Work out the finished part from the listing and answer in its coordinate system (mm). Face numbers are marked on the shaded views. A direction names the side the tool comes from. Give positions to 0.01 mm unless a question says otherwise; leave off trailing zeros. Loops run counter-clockwise (first coordinate to the right, second up) from the corner with the lowest first, then second, coordinate; pieces in that order, holes last. Notation, with made-up numbers: (-16.75, 33.25) - (19.25, 33.25) arc R18 cw to (19.25, 39.25) - close; hole circle Ø3 at (-24, 41). An arc over 180 degrees is marked (long way). One line per question, with ' | ' between items. Start each with the question number.
1. Section A-A (z = -5) is taken. Determine the outline of the cut face in (x, y), plus the area to 3 significant figures.
2. Which of the six approach directions +Z, -Z, +X, -X, +Y, -Y give full straight-line access (tool end or side, diameter ignored) to the marked faces 4 and 5?
3. Find the intervals of material crossed by line 1 (X direction, y = 50, z = 4); line 2 (Y direction, x = 61.5, z = -4.25); line 3 (Y direction, x = -62, z = 1.5), in increasing order.
4. This flat-tipped pin is pushed along its axis until it touches: pin 1 (11 mm diameter, centred on x = -61.5, y = -50, fed in from -Z). Where does it stop, or does it pass through?
5. Section D-D (z = 5.25) is taken. Determine the outline of the cut face in (x, y), plus the area to 3 significant figures.
6. For a pull along X with two mould halves and no side action, classify the marked faces 1, 2 and 3 as released by +X, released by -X, zero draft, split by the parting line, or undercut.
7. Section B-B (x = -61.5) is taken. Determine the outline of the cut face in (y, z), plus the area to 3 significant figures.
8. Section C-C (y = -19) is taken. Determine the outline of the cut face in (x, z), plus the area to 3 significant figures.
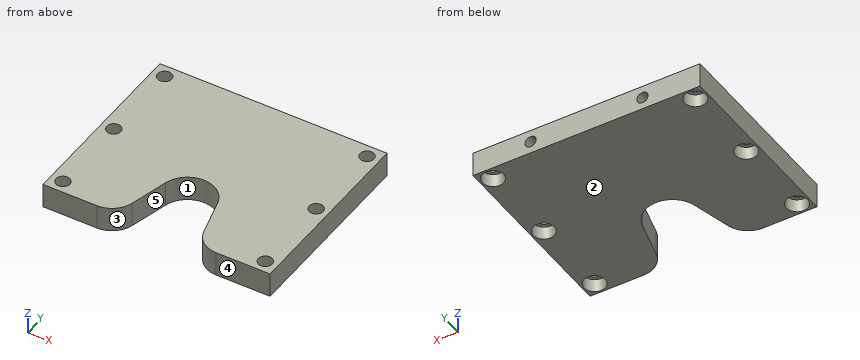
from build123d import *

# Parameters (mm, degrees)
CROQUIS1_R                = 4.25
SALIENTE_EXTRUIR1_DEPTH   = 7.5
CROQUIS2_R                = 6.5
CORTAR_EXTRUIR1_DEPTH     = 8
TALADRO_ROSCADO_M81_D     = 6.8
TALADRO_ROSCADO_M81_DEPTH = 20
TALADRO_ROSCADO_M81_TIP   = 2.042926105


with BuildPart() as part:
    # Croquis1 → Saliente-Extruir1 (new body, symmetric)
    with BuildSketch(Plane.XY):
        with BuildLine():
            Line((69, -57.5), (36.3, -57.5))
            ThreePointArc((36.3, -57.5), (27.113751898, -54.358028749), (21.775894122, -46.248379441))
            Line((21.775894122, -46.248379441), (15.782861721, -23.026761008))
            ThreePointArc((15.782861721, -23.026761008), (0, -10.8), (-15.782861721, -23.026761008))
            Line((-15.782861721, -23.026761008), (-21.775894122, -46.248379441))
            ThreePointArc((-21.775894122, -46.248379441), (-27.113751898, -54.358028749), (-36.3, -57.5))
            Line((-36.3, -57.5), (-69, -57.5))
            Line((-69, -57.5), (-69, 57.5))
            Line((-69, 57.5), (69, 57.5))
            Line((69, 57.5), (69, -57.5))
        make_face()
        with Locations((-61.5, 50)):
            Circle(CROQUIS1_R, mode=Mode.SUBTRACT)
        with Locations((-61.5, 0)):
            Circle(CROQUIS1_R, mode=Mode.SUBTRACT)
        with Locations((-61.5, -50)):
            Circle(CROQUIS1_R, mode=Mode.SUBTRACT)
        with Locations((61.5, 50)):
            Circle(CROQUIS1_R, mode=Mode.SUBTRACT)
        with Locations((61.5, 0)):
            Circle(CROQUIS1_R, mode=Mode.SUBTRACT)
        with Locations((61.5, -50)):
            Circle(CROQUIS1_R, mode=Mode.SUBTRACT)
    extrude(amount=SALIENTE_EXTRUIR1_DEPTH, both=True)

    # Croquis2 → Cortar-Extruir1 (cut)
    with BuildSketch(Plane(origin=(0, 0, -7.5), x_dir=(-1, 0, 0), z_dir=(0, 0, -1))):
        with Locations((-61.5, 50)):
            Circle(CROQUIS2_R)
        with Locations((-61.5, 0)):
            Circle(CROQUIS2_R)
        with Locations((-61.5, -50)):
            Circle(CROQUIS2_R)
        with Locations((61.5, 50)):
            Circle(CROQUIS2_R)
        with Locations((61.5, 0)):
            Circle(CROQUIS2_R)
        with Locations((61.5, -50)):
            Circle(CROQUIS2_R)
    extrude(amount=-CORTAR_EXTRUIR1_DEPTH, mode=Mode.SUBTRACT)

    # Taladro roscado M81
    with Locations(Plane(origin=(0, 57.5, 0), x_dir=(-1, 0, 0), z_dir=(0, 1, 0))):
        with Locations((34, 0), (-34, 0)):
            Hole(TALADRO_ROSCADO_M81_D / 2, depth=TALADRO_ROSCADO_M81_DEPTH)
            with Locations((0, 0, -(TALADRO_ROSCADO_M81_DEPTH + TALADRO_ROSCADO_M81_TIP / 2))):  # 118° drill point
                Cone(0, TALADRO_ROSCADO_M81_D / 2, TALADRO_ROSCADO_M81_TIP, mode=Mode.SUBTRACT)


solid = part.part
Conclusion:
1) outline: (-69, -57.5) - (-36.3, -57.5) arc R15 ccw to (-21.78, -46.25) - (-15.78, -23.03) arc R16.3 cw to (15.78, -23.03) - (21.78, -46.25) arc R15 ccw to (36.3, -57.5) - (69, -57.5) - (69, 57.5) - (-69, 57.5) - close; hole circle Ø13 at (-61.5, -50); hole circle Ø13 at (-61.5, 0); hole circle Ø13 at (-61.5, 50); hole circle Ø13 at (61.5, -50); hole circle Ø13 at (61.5, 0); hole circle Ø13 at (61.5, 50) | area: 13,300 mm²
2) face 4: +Z, -Z, +X, -X, -Y | face 5: +Z, -Z, -Y
3) line 1: -69 to -65.75, -57.25 to 57.25, 65.75 to 69 | line 2: -57.5 to -56.5, -43.5 to -6.5, 6.5 to 43.5, 56.5 to 57.5 | line 3: -57.5 to -54.22, -45.78 to -4.22, 4.22 to 45.78, 54.22 to 57.5
4) pin 1: z = 0.5
5) outline: (-69, -57.5) - (-36.3, -57.5) arc R15 ccw to (-21.78, -46.25) - (-15.78, -23.03) arc R16.3 cw to (15.78, -23.03) - (21.78, -46.25) arc R15 ccw to (36.3, -57.5) - (69, -57.5) - (69, 57.5) - (-69, 57.5) - close; hole circle Ø8.5 at (-61.5, -50); hole circle Ø8.5 at (-61.5, 0); hole circle Ø8.5 at (-61.5, 50); hole circle Ø8.5 at (61.5, -50); hole circle Ø8.5 at (61.5, 0); hole circle Ø8.5 at (61.5, 50) | area: 13,800 mm²
6) face 1: undercut | face 2: zero draft | face 3: undercut
7) outline: (-57.5, -7.5) - (-56.5, -7.5) - (-56.5, 0.5) - (-54.25, 0.5) - (-54.25, 7.5) - (-57.5, 7.5) - close; (-45.75, 0.5) - (-43.5, 0.5) - (-43.5, -7.5) - (-6.5, -7.5) - (-6.5, 0.5) - (-4.25, 0.5) - (-4.25, 7.5) - (-45.75, 7.5) - close; (4.25, 0.5) - (6.5, 0.5) - (6.5, -7.5) - (43.5, -7.5) - (43.5, 0.5) - (45.75, 0.5) - (45.75, 7.5) - (4.25, 7.5) - close; (54.25, 0.5) - (56.5, 0.5) - (56.5, -7.5) - (57.5, -7.5) - (57.5, 7.5) - (54.25, 7.5) - close | area: 1,230 mm²
8) outline: (-69, -7.5) - (-14.14, -7.5) - (-14.14, 7.5) - (-69, 7.5) - close; (14.14, -7.5) - (69, -7.5) - (69, 7.5) - (14.14, 7.5) - close | area: 1,650 mm²
